For this review, use the dimensioned drawing (mm, ordinates from the lowest corner) and the shaded views. Round coordinates to 2 decimals unless told otherwise and drop trailing zeros. Loops run counter-clockwise (first coordinate to the right, second up) from the corner with the lowest first, then second, coordinate; pieces in that order, holes last. Notation, with made-up numbers: M -3,8 L 42,8 A15 cw 42,14 Z; hole C 42.25,81 d4. An arc over 180 degrees is marked long. Use a Markdown table: item, result. Add a question column.
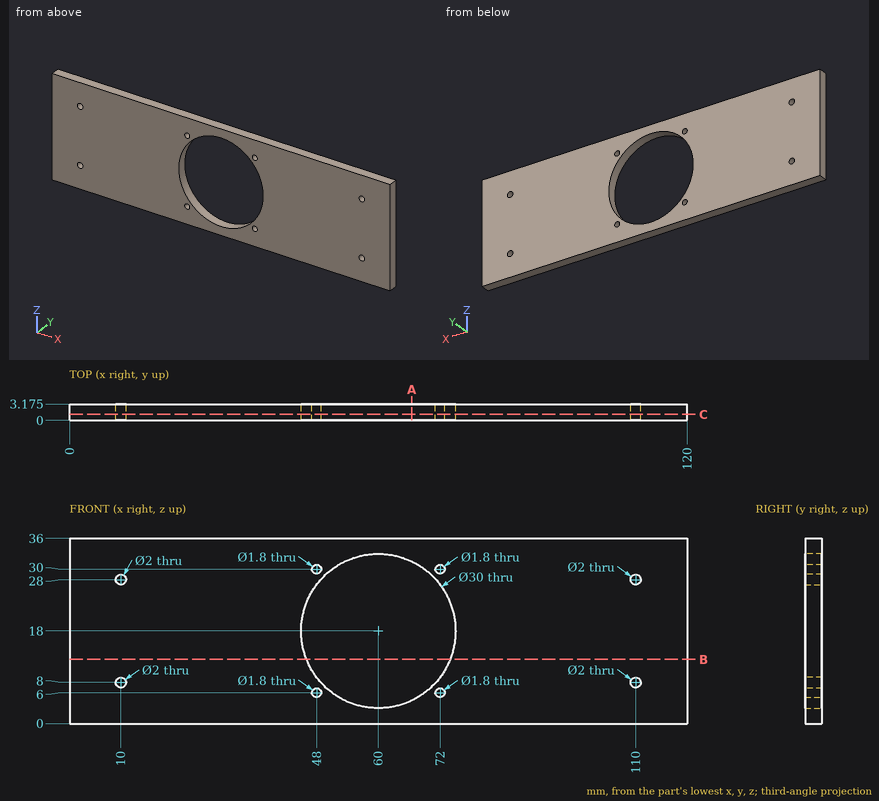
(1) Consider section A-A, the plane x = 66.5. Give the boundary of the cut face in (y, z) (1 decimal), then the cut area to 3 significant figures.
(2) Consider section C-C, the plane y = 1.15. Give the number of separate pieces and of enclosed holes in the cut face, then the cut area to 3 significant figures.
(3) To check wall thickness, follow probe 1 along Z at (x, y) = (10, 2.15); probe 2 along Z at (x, y) = (72, 1.65); probe 3 along X at (y, z) = (3.05, 18). State the ranges of each line that lie inside material, in increasing order.
(4) Consider section B-B, the plane z = 12.5. Give the boundary of the cut face in (x, y) (3 decimals).
(5) Insertion check: pin 1 Ø1.5 at (y, z) = (2, 18.5) entering from -X. The pin has a flat end and moves straight along its axis. Give the tip position at first contact, or say it passes through.
Found:
| question | item | result |
|---|---|---|
| 1 | outline | M 0,0 L 3.2,0 L 3.2,4.5 L 0,4.5 Z; M 0,31.5 L 3.2,31.5 L 3.2,36 L 0,36 Z |
| 1 | area | 28.5 mm^2 |
| 2 | separate pieces | 1 |
| 2 | enclosed holes | 9 |
| 2 | area | 3,590 mm^2 |
| 3 | probe 1 | z = 0 to 7, 9 to 27, 29 to 36 |
| 3 | probe 2 | z = 0 to 5.1, 6.9 to 9, 27 to 29.1, 30.9 to 36 |
| 3 | probe 3 | x = 0 to 45, 75 to 120 |
| 4 | outline | M 0,0 L 46.045,0 L 46.045,3.175 L 0,3.175 Z; M 73.955,0 L 120,0 L 120,3.175 L 73.955,3.175 Z |
| 5 | pin 1 | stops at x = 0 |
